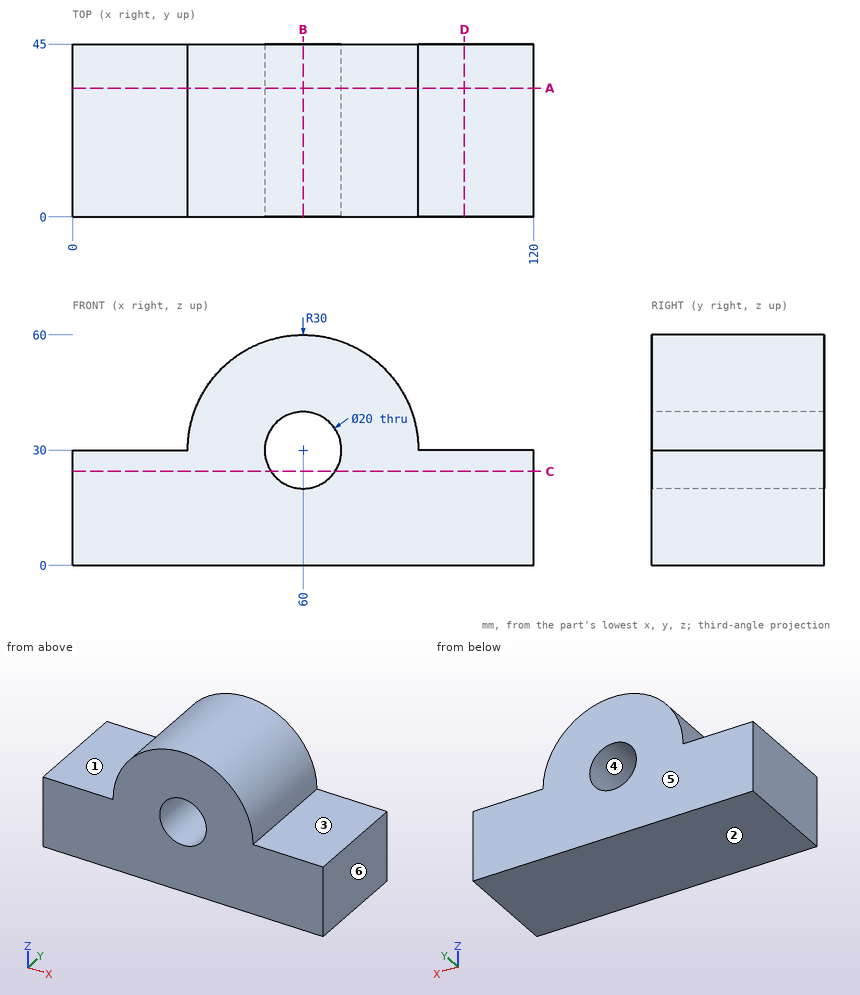
Study the drawing (mm; zero at the part's minimum x, y, z) and answer. A direction names the side the tool comes from. Coordinates: 2 decimals unless noted, no trailing zeros. Loops run counter-clockwise (first coordinate to the right, second up) from the corner with the lowest first, then second, coordinate; pieces in that order, holes last. Notation, with made-up numbers: M 16,78.25 L 40,78.25 A23 cw 40,112.25 Z; hole C -7.75,-34 d1. An arc over 180 degrees is marked long. Answer in a Markdown table with one row per item. Add a question column.
1. The mould has two halves that part along X. Classify the marked faces 4, 5 and 6: pulls with the +X half, pulls with the -X half, needs draft (parallel to the pull), parting line crosses it, or undercut.
2. Find section A-A, the plane y = 33.5. Write down the section's boundary in (x, z).
3. Consider L1, parallel to Z at x = 60, y = 19; L2, parallel to X at y = 25, z = 38; L3, parallel to Z at x = 63, y = 35. Determine where each line is inside the solid, lowest interval first.
4. Find section B-B, the plane x = 60. Write down the section's boundary in (y, z).
5. Find section C-C, the plane z = 24.5. Write down the section's boundary in (x, y), then the cut area to 3 significant figures.
6. A tool of negligible diameter and unlimited length cuts with its end or side. For the marked faces 1, 2 and 3, from which of +Z, -Z, +X, -X, +Y, -Y can it reach the whole face along a straight path? Write none if from no direction.
7. Find section D-D, the plane x = 102. Write down the section's boundary in (y, z), then the cut area to 3 significant figures.
8. Flat-ended cylindrical pins translate along their axes: P1, Ø4, axis at y = 20.5, z = 41.5, coming from the -X side; P2, Ø1.5, axis at x = 53, y = 19, coming from the +Z side; P3, Ø6, axis at x = 103.5, y = 21, coming from the +Z side. Find the tip coordinate at first contact, or state that the pin passes through.
Reported:
| question | item | result |
|---|---|---|
| 1 | face 4 | undercut |
| 1 | face 5 | needs draft |
| 1 | face 6 | pulls with the +X half |
| 2 | outline | M 0,0 L 120,0 L 120,30 L 90,30 A30 ccw 30,30 L 0,30 Z; hole C 60,30 d20 |
| 3 | L1 | z = 0 to 20, 40 to 60 |
| 3 | L2 | x = 31.09 to 54, 66 to 88.91 |
| 3 | L3 | z = 0 to 20.46, 39.54 to 59.85 |
| 4 | outline | M 0,0 L 45,0 L 45,20 L 0,20 Z; M 0,40 L 45,40 L 45,60 L 0,60 Z |
| 5 | outline | M 0,0 L 51.65,0 L 51.65,45 L 0,45 Z; M 68.35,0 L 120,0 L 120,45 L 68.35,45 Z |
| 5 | area | 4,650 mm^2 |
| 6 | face 1 | +Z, -X, +Y, -Y |
| 6 | face 2 | -Z, +X, -X, +Y, -Y |
| 6 | face 3 | +Z, +X, +Y, -Y |
| 7 | outline | M 0,0 L 45,0 L 45,30 L 0,30 Z |
| 7 | area | 1,350 mm^2 |
| 8 | P1 | stops at x = 31.54 |
| 8 | P2 | stops at z = 59.34 |
| 8 | P3 | stops at z = 30 |
